The drawing under review shows one solid part. Ordinate dimensions are in mm from its lowest x, y, z. A direction names the side the tool comes from. Coordinates: 2 decimals unless noted, no trailing zeros. Order: outer loops, then holes, each group sorted by start corner. A loop starts at its lowest first (then second) coordinate and runs counter-clockwise, first axis right, second up.
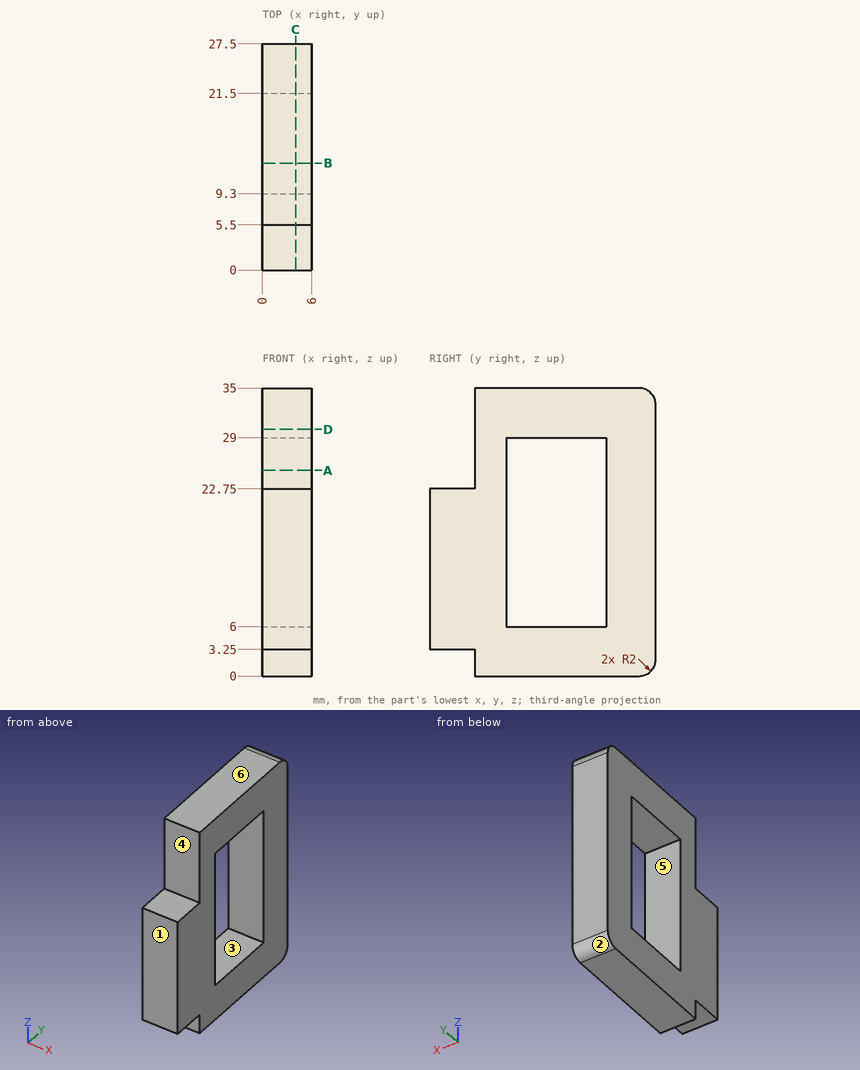
1. To check wall thickness, follow L1, parallel to Z at x = 4.85, y = 13.75; L2, parallel to Y at x = 3.05, z = 12; L3, parallel to Y at x = 5.15, z = 24. State the ranges of each line that lie inside material, in increasing order.
Answer below:
L1: z = 0 to 6, 29 to 35
L2: y = 0 to 9.3, 21.5 to 27.5
L3: y = 5.5 to 9.3, 21.5 to 27.5
2. Take a section at D-D, the plane z = 30. Give the boundary of the cut face in (x, y).
Answer below:
outline: (0, 5.5) - (6, 5.5) - (6, 27.5) - (0, 27.5) - close
3. Take a section at C-C, the plane x = 4.05. Give the boundary of the cut face in (y, z), plus the area to 3 significant figures.
Answer below:
outline: (0, 3.25) - (5.5, 3.25) - (5.5, 0) - (25.5, 0) arc R2 ccw to (27.5, 2) - (27.5, 33) arc R2 ccw to (25.5, 35) - (5.5, 35) - (5.5, 22.75) - (0, 22.75) - close; hole (9.3, 6) - (21.5, 6) - (21.5, 29) - (9.3, 29) - close
area: 595 mm2
4. Take a section at A-A, the plane z = 25. Give the boundary of the cut face in (x, y).
Answer below:
outline: (0, 5.5) - (6, 5.5) - (6, 9.3) - (0, 9.3) - close; (0, 21.5) - (6, 21.5) - (6, 27.5) - (0, 27.5) - close
5. Clearance check with flat-ended pins moving along their axes: pin 1 Ø3 at (x, y) = (3, 2.5) entering from -Z; pin 2 Ø1.6 at (x, y) = (1.5, 3) entering from +Z; pin 3 Ø3.5 at (x, z) = (3.5, 1) entering from -Y. State where each tip first meets the part, or that it passes through.
Answer below:
pin 1: stops at z = 3.25
pin 2: stops at z = 22.75
pin 3: stops at y = 5.5
6. Machinability: for the marked faces 4, 5 and 6, which of the approach directions +Z, -Z, +X, -X, +Y, -Y give a long, thin tool a straight path to every point of the face, cutting with its end or side? Answer none if there is none.
Answer below:
face 4: +Z, +X, -X, -Y
face 5: +X, -X
face 6: +Z, +X, -X, +Y, -Y
7. The part is to be moulded in two halves that separate along Z. For the marked faces 1, 2 and 3, say which applies: +Z half, -Z half, draft (parallel to the pull), parting line (faces both ways), or undercut.
Answer below:
face 1: draft
face 2: -Z half
face 3: undercut
8. Take a section at B-B, the plane y = 13. Give the boundary of the cut face in (x, z).
Answer below:
outline: (0, 0) - (6, 0) - (6, 6) - (0, 6) - close; (0, 29) - (6, 29) - (6, 35) - (0, 35) - close
